```python
from build123d import *

# Parameters (mm, degrees)
CHAMFER1_SIZE = 1


with BuildPart() as part:
    # Sketch3 → Revolve2 (revolve)
    with BuildSketch(Plane(origin=(0, 0, 0), x_dir=(0, 0, -1), z_dir=(1, 0, 0))):
        Polygon((-29, -21.25), (-29, -14.25), (-27, -14.25), (-27, -12.25), (-30, -12.25), (-30, 12.75), (-27, 12.75), (-27, 14.75), (-29, 14.75), (-29, 21.25), (-32.5, 21.25), (-32.5, -21.25), align=None)
    revolve(axis=Axis((0, -21.25, 0), (0, 1, 0)))

    # Chamfer1
    chamfer1_edges = [part.edges().sort_by_distance(p)[0] for p in [
        (0, -21.25, -32.5),
    ]]
    chamfer(chamfer1_edges, length=CHAMFER1_SIZE)


solid = part.part
```
Input: part model. Units: mm. Frame: model coordinates. A direction names the side the tool comes from. Coordinates: 2 decimals unless noted, no trailing zeros. Loops run counter-clockwise (first coordinate to the right, second up) from the corner with the lowest first, then second, coordinate; pieces in that order, holes last. Notation, with made-up numbers: (-17, 50) -> (30, 50) arc R22 cw to (30, 68) -> close; hole circle Ø4 at (79.5, 12). An arc over 180 degrees is marked (long way). Use a Markdown table: item, result.
1) Material intervals for line 1 along X through (y, z) = (16.5, 0); line 2 along X through (y, z) = (1, 0); line 3 along Y through (x, z) = (14.5, 23), sorted ascending. Write a range as from..to.
Results found:
| item | result |
|---|---|
| line 1 | x = -32.5..-29, 29..32.5 |
| line 2 | x = -32.5..-30, 30..32.5 |
| line 3 | y = -14.25..-12.25, 12.75..14.75 |
2) Access query for faces 1 (the cylindrical face through (1.32, 0.43, -29.97)), 2 (the cylindrical face through (-25.73, 18.05, 13.38)), 3 (the flat face through (-26, -14.25, 8)), 4 (the cylindrical face through (-26.36, 13.76, -5.85)). Directions: +Z, -Z, +X, -X, +Y, -Y. A direction counts if a zero-diameter tool reaches every point of the face in a straight line with its end or side. Return the directions, or none.
Results found:
| item | result |
|---|---|
| face 1 | none |
| face 2 | +Y |
| face 3 | -Y |
| face 4 | +Y, -Y |
3) Cut plane B-B (z = 0). Return the cut outline in (x, y).
Results found:
| item | result |
|---|---|
| outline | (-32.5, -20.25) -> (-31.5, -21.25) -> (-29, -21.25) -> (-29, -14.25) -> (-27, -14.25) -> (-27, -12.25) -> (-30, -12.25) -> (-30, 12.75) -> (-27, 12.75) -> (-27, 14.75) -> (-29, 14.75) -> (-29, 21.25) -> (-32.5, 21.25) -> close; (27, -14.25) -> (29, -14.25) -> (29, -21.25) -> (31.5, -21.25) -> (32.5, -20.25) -> (32.5, 21.25) -> (29, 21.25) -> (29, 14.75) -> (27, 14.75) -> (27, 12.75) -> (30, 12.75) -> (30, -12.25) -> (27, -12.25) -> close |
4) Contact query for flat-ended pins moving along their axis: pin 1 (3 mm diameter, centred on x = -20, y = 4, fed in from -Z); pin 2 (1 mm diameter, centred on x = -24.5, z = -2.5, fed in from -Y); pin 3 (1 mm diameter, centred on x = -15.5, y = -6.5, fed in from +Z); pin 4 (8 mm diameter, centred on y = 9, z = 15, fed in from -X). Output: stop coordinate, or through.
Results found:
| item | result |
|---|---|
| pin 1 | stops at z = -26.72 |
| pin 2 | passes through |
| pin 3 | stops at z = 28.83 |
| pin 4 | stops at x = -30.58 |
5) Cut plane A-A (x = 0). Return the cut outline in (y, z).
Results found:
| item | result |
|---|---|
| outline | (-21.25, -31.5) -> (-20.25, -32.5) -> (21.25, -32.5) -> (21.25, -29) -> (14.75, -29) -> (14.75, -27) -> (12.75, -27) -> (12.75, -30) -> (-12.25, -30) -> (-12.25, -27) -> (-14.25, -27) -> (-14.25, -29) -> (-21.25, -29) -> close; (-21.25, 29) -> (-14.25, 29) -> (-14.25, 27) -> (-12.25, 27) -> (-12.25, 30) -> (12.75, 30) -> (12.75, 27) -> (14.75, 27) -> (14.75, 29) -> (21.25, 29) -> (21.25, 32.5) -> (-20.25, 32.5) -> (-21.25, 31.5) -> close |
6) Pull-direction query (Y, two-part tool) for faces 5 (the flat face through (-5, 21.25, 29)), 6 (the flat face through (-26, -21.25, 14)), 7 (the flat face through (11, -12.25, 25)), 8 (the cylindrical face through (-26.36, -13.24, -5.85)); classes: released by +Y, released by -Y, zero draft, split by the parting line, or undercut.
Results found:
| item | result |
|---|---|
| face 5 | released by +Y |
| face 6 | released by -Y |
| face 7 | undercut |
| face 8 | zero draft |
7) Cut plane C-C (y = 6.5). Return the cut outline in (x, z).
Results found:
| item | result |
|---|---|
| outline | circle Ø65 at (0, 0); hole circle Ø60 at (0, 0) |
